Autodesk Inventor part; units mm, degrees
ref_plane "YZ Plane" through (0, 0, 0) normal (1, 0, 0) x (0, 1, 0)
ref_plane "XZ Plane" through (0, 0, 0) normal (0, 1, 0) x (-1, 0, 0)
ref_plane "XY Plane" through (0, 0, 0) normal (0, 0, 1) x (1, 0, 0)
sketch "Sketch1" plane through (0, 0, 0) normal (0, 0, 1) x (1, 0, 0)
  line L0 (130, 90) -> (-130, -90) construction
  line L1 (-130, 90) -> (130, -90) construction
  circle A0 centre (-105, 65) radius 16
  circle A1 centre (105, 65) radius 16
  circle A2 centre (105, -65) radius 16
  circle A3 centre (-105, -65) radius 16
  line L2 (0, -68.1117) -> (0, -128.2653) construction
  line L3 (-8, -68.1117) -> (-8, -90)
  line L4 (8, -90) -> (8, -68.1117)
  arc A4 (8, -68.1117) -> (-8, -68.1117) centre (0, -68.1117) ccw
  line L5 (138.2624, 0) -> (110, 0) construction
  line L6 (130, 4) -> (110, 4)
  line L7 (110, -4) -> (130, -4)
  arc A5 (110, 4) -> (110, -4) centre (110, 0) ccw
  line L8 (-67.4567, 0.3936) -> (51.9271, 0.3936) construction
  line L9 (0, -23.6129) -> (0, 33.7533) construction
  line L10 (-8, 68.899) -> (-8, 90)
  line L11 (8, 90) -> (8, 68.899)
  arc A6 (-8, 68.899) -> (8, 68.899) centre (0, 68.899) ccw
  line L12 (-130, -90) -> (-8, -90)
  line L13 (8, -90) -> (130, -90)
  line L14 (130, -90) -> (130, -4)
  line L15 (130, 4) -> (130, 90)
  line L16 (130, 90) -> (8, 90)
  line L17 (-8, 90) -> (-130, 90)
  line L18 (-130, 4) -> (-110, 4)
  line L19 (-110, -4) -> (-130, -4)
  arc A7 (-110, -4) -> (-110, 4) centre (-110, 0) ccw
  line L20 (-130, 90) -> (-130, 4)
  line L21 (-130, -4) -> (-130, -90)
  point P0 (0, 0)
  point P1 (4, -128.8323)
  point P2 (0, -98.1885)
  point P3 (124.1312, 0)
  point P4 (4, -87.7077)
  point P5 (130, 0)
  point P6 (-4, 128.8323)
  point P7 (4, 129.6196)
  dimension "d2" = 32
  dimension "d3" = 105
  dimension "d5" = 65
  dimension "d6" = 105
  dimension "d7" = 65
  dimension "d9" = 8
  dimension "d10" = 20
  dimension "d11" = 20
  dimension "d24" = 8
  dimension "d25" = 101
  dimension "d26" = 97
  dimension "d27" = 97
  dimension "d28" = 65
  dimension "d29" = 65
  dimension "d30" = 0
  dimension "d31" = 4
  dimension "d32" = 4
  dimension "d33" = 260
  dimension "d34" = 260
  dimension "d35" = 180
  dimension "d36" = 180
extrude "Extrusion1" add sketch "Sketch1" along normal blind 16
sketch "Sketch2" plane through (0, 0, 16) normal (0, 0, 1) x (1, 0, 0)
  circle A0 centre (35, 0) radius 2.5
  point P0 (0, 0)
  dimension "d14" = 5
  dimension "d15" = 35
extrude "Extrusion2" cut sketch "Sketch2" against normal blind 12
sketch "Sketch3" plane through (0, 0, 16) normal (0, 0, 1) x (1, 0, 0)
  circle A0 centre (0, 0) radius 17.5
  dimension "d18" = 35
extrude "Extrusion3" cut sketch "Sketch3" against normal blind 10
pattern_circular "Circular Pattern1" count 4 over 360 about axis through (0, 0, 16) along (0, 0, -1) of "Extrusion2"
properties part number "Base superior da ferramenta"
Build history of the part. All positions in model axes, mm. A direction names the side the tool comes from. Give positions to 0.01 mm unless a question says otherwise; leave off trailing zeros. Order: outer loops, then holes, each group sorted by start corner. A loop starts at its lowest first (then second) coordinate and runs counter-clockwise, first axis right, second up. Notation, with made-up numbers: M -11,-22.5 L 19,-22.5 A10 cw 19,-17.5 Z; hole C 66.25,-5 d11. An arc over 180 degrees is marked long. Write item = value, one per line. Start each with the question number.
(1) Two-plate mould, pull along Y, no slides. Class faces 1 (the flat face through (-8, -79, 8)), 2 (the cylindrical face through (106, 0, 8)), 3 (the flat face through (68, -90, 8)), 4 (the cylindrical face through (-106, 0, 8)): released by +Y, released by -Y, zero draft, split by the parting line, or undercut.
(2) Slice it at C-C on y = -65. Write the cut outline in (x, z), plus the area to 3 significant figures.
(3) Slice it at A-A on z = 9.5. State how many separate pieces and enclosed holes the cut face has, plus the area to 3 significant figures.
(4) Which spindle directions (+Z, -Z, +X, -X, +Y, -Y) get a long thin tool onto all of the face, cutting with end or side? Do faces 5 (the flat face through (-2, -19, 16)), 6 (the flat face through (120, -4, 8)), 7 (the cylindrical face through (0.96, 37.31, 10.08)). Say none if no direction does.
(5) Slice it at D-D on y = 11. Write the cut outline in (x, z).
(6) Slice it at B-B on x = 95. Write the cut outline in (y, z), plus the area to 3 significant figures.
(7) Pin check, flat tips, straight feed: pin 1 Ø4.5 at (x, y) = (0, -35) entering from -Z; pin 2 Ø4 at (x, y) = (0, 35) entering from +Z; pin 3 Ø17.5 at (x, y) = (-2, 6.5) entering from +Z. Stop position of each tip, or through.
(8) Probe L1, parallel to Y at x = 105, z = 6.75; L2, parallel to X at y = -35.5, z = 4.75; L3, parallel to Y at x = 35, z = 9.25. List the from-to ranges inside material, lowest first. Write a range as [from, to].
Responses:
q1.face_1 = zero draft
q1.face_2 = undercut
q1.face_3 = released by -Y
q1.face_4 = undercut
q2.outline = M -130,0 L -121,0 L -121,16 L -130,16 Z; M -89,0 L -7.37,0 L -7.37,16 L -89,16 Z; M 7.37,0 L 89,0 L 89,16 L 7.37,16 Z; M 121,0 L 130,0 L 130,16 L 121,16 Z
q2.area = 2,900 mm2
q3.separate_pieces = 1
q3.enclosed_holes = 9
q3.area = 41,300 mm2
q4.face_5 = +Z, +X, -X, +Y, -Y
q4.face_6 = +Z, -Z, +X
q4.face_7 = +Z
q5.outline = M -130,0 L 130,0 L 130,16 L 13.61,16 L 13.61,6 L -13.61,6 L -13.61,16 L -130,16 Z
q6.outline = M -90,0 L -77.49,0 L -77.49,16 L -90,16 Z; M -52.51,0 L 52.51,0 L 52.51,16 L -52.51,16 Z; M 77.49,0 L 90,0 L 90,16 L 77.49,16 Z
q6.area = 2,080 mm2
q7.pin_1 = 0
q7.pin_2 = 4
q7.pin_3 = 6
q8.L1 = [-90, -81], [-49, 49], [81, 90]
q8.L2 = [-130, -2.45], [2.45, 130]
q8.L3 = [-90, -2.5], [2.5, 90]
